Could you check a few things on this model? Use its own coordinates, in mm. Give positions to 0.01 mm unless a question says otherwise; leave off trailing zeros. Loops run counter-clockwise (first coordinate to the right, second up) from the corner with the lowest first, then second, coordinate; pieces in that order, holes last. Notation, with made-up numbers: M 21,82 L 63,82 A28 ccw 63,114 Z; hole C -30,53 d3. An arc over 180 degrees is marked long. Answer in a Markdown table with one row per item. Add a question column.
1. I need wall thicknesses on line 1 along X through (y, z) = (638.5, -42.5); line 2 along Z through (x, y) = (16.5, 1338); line 3 along X through (y, z) = (1257, -43). Which ranges of each line are inside material? Lowest first, please. Write a range as from..to.
2. If we section it at B-B on x = 44: List the corners of the cut face in (y, z) for me.
3. I'm going to push flat-ended pins straight in: pin 1 Ø6 at (x, y) = (50, 1166) entering from -Z; pin 2 Ø1 at (x, y) = (53, 952.5) entering from -Z; pin 3 Ø1.5 at (x, y) = (41.5, 790) entering from -Z. Where does each tip first touch, or does it pass through?
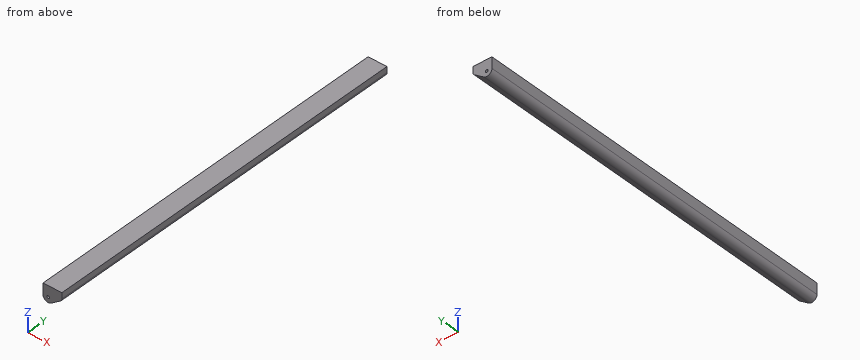
```python
from build123d import *

# Parameters (mm, degrees)
SKETCH1_R           = 4.7625
BOSS_EXTRUDE1_DEPTH = 1397


with BuildPart() as part:
    # Sketch1 → Boss-Extrude1 (new body)
    with BuildSketch(Plane(origin=(0, 0, 0), x_dir=(1, 0, 0), z_dir=(0, 1, 0))):
        with BuildLine():
            ThreePointArc((29.976631112, 55.849090528), (10.253688918, 57.141800456), (0, 40.244244084))
            Line((0, 40.244244084), (0, 0))
            Line((0, 0), (69.85, 0))
            Line((69.85, 0), (69.85, 21.318255517))
            ThreePointArc((69.85, 21.318255517), (68.415037581, 27.182462905), (64.434420742, 31.721486479))
            Line((64.434420742, 31.721486479), (29.976631112, 55.849090528))
        make_face()
        with Locations(Location((19.05, 40.244244084, 0), (0, 0, 270))):
            Circle(SKETCH1_R, mode=Mode.SUBTRACT)
    extrude(amount=BOSS_EXTRUDE1_DEPTH)


solid = part.part
```
Results:
| question | item | result |
|---|---|---|
| 1 | line 1 | 0.13..14.86, 23.24..49.04 |
| 1 | line 2 | -59.12..-44.27, -36.22..0 |
| 1 | line 3 | 0.2..15.17, 22.93..48.33 |
| 2 | outline | M 0,-46.03 L 1397,-46.03 L 1397,0 L 0,0 Z |
| 3 | pin 1 | z = -43.93 |
| 3 | pin 2 | z = -40.08 |
| 3 | pin 3 | z = -48.31 |
